Here's how the part is built. I have some questions about the finished solid (model axes, mm). Face numbers are marked on the shaded views. A direction names the side the tool comes from. Coordinates: 2 decimals unless noted, no trailing zeros. Write each loop counter-clockwise with the first axis right and the second up, starting at its lowest first coordinate (ties: lowest second). Pieces come first, ordered by that corner, then holes.
(1) For pin 1 Ø4 at (x, z) = (-41, 31) entering from +Y; pin 2 Ø2.5 at (x, y) = (39.5, -1) entering from +Z; pin 3 Ø5.5 at (y, z) = (4.5, 50.5) entering from -X, each with a flat end and sliding along its axis, tell me the tip position at first contact or that it passes through.
(2) Imagine slicing it at B-B, the plane z = 27.5. List the corners of the cut face in (x, y) for me.
(3) Which directions (+Z, -Z, +X, -X, +Y, -Y) give clear straight access to the entire face, cutting with the end or side of a thin tool? Please do the marked faces 1, 2, 3 and 4.
(4) Imagine slicing it at A-A, the plane y = 4.5. List the corners of the cut face in (x, z) for me.
(5) Imagine slicing it at C-C, the plane x = -28.5. List the corners of the cut face in (y, z) for me.
(6) Please list where these lines run through material, in increasing order: probe 1 along Z at (x, y) = (13.5, -5); probe 2 along X at (y, z) = (-6, 5.5); probe 3 along Y at (x, z) = (-12, 51).
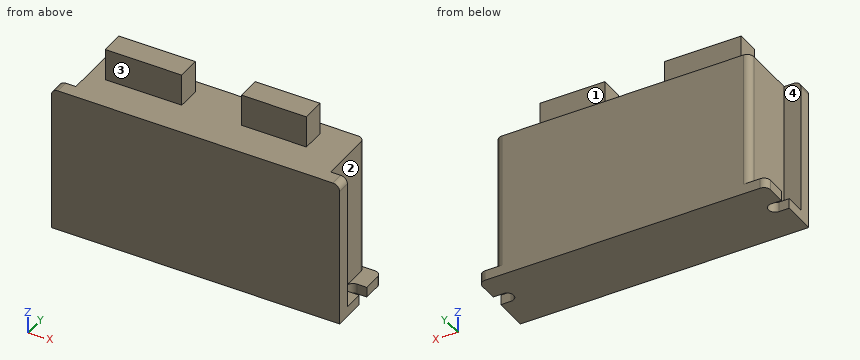
```python
from build123d import *

# Parameters (mm, degrees)
SKETCH1_W           = 86
SKETCH1_H           = 21.5
BOSS_EXTRUDE1_DEPTH = 43.75
SKETCH2_W           = 5
SKETCH2_H           = 17.5
CUT_EXTRUDE1_DEPTH  = 40.75
CUT_EXTRUDE2_DEPTH  = 63.278607884
FILLET1_R           = 2
SKETCH4_W           = 22.8
SKETCH4_H           = 7
SKETCH4_W_2         = 19.4
BOSS_EXTRUDE2_DEPTH = 9.5


with BuildPart() as part:
    # Sketch1 → Boss-Extrude1 (new body)
    with BuildSketch(Plane.XY):
        Rectangle(SKETCH1_W, SKETCH1_H)
    extrude(amount=BOSS_EXTRUDE1_DEPTH)

    # Sketch2 → Cut-Extrude1 (cut)
    with BuildSketch(Plane.XY.offset(43.75)):
        with Locations((-40.5, 2)):
            Rectangle(SKETCH2_W, SKETCH2_H)
        with Locations((40.5, 2)):
            Rectangle(SKETCH2_W, SKETCH2_H)
    extrude(amount=-CUT_EXTRUDE1_DEPTH, mode=Mode.SUBTRACT)

    # Sketch3 → Cut-Extrude2 (cut, through all)
    with BuildSketch(Plane(origin=(0, 0, 0), x_dir=(-1, 0, 0), z_dir=(0, 0, -1))):
        with BuildLine():
            Line((40, 3.25), (47.671145092, 3.25))
            ThreePointArc((47.671145092, 3.25), (49.671145092, 1.25), (47.671145092, -0.75))
            Line((47.671145092, -0.75), (40, -0.75))
            ThreePointArc((40, -0.75), (38, 1.25), (40, 3.25))
        make_face()
        with BuildLine():
            Line((-40, 3.25), (-47.671145092, 3.25))
            ThreePointArc((-47.671145092, 3.25), (-49.671145092, 1.25), (-47.671145092, -0.75))
            Line((-47.671145092, -0.75), (-40, -0.75))
            ThreePointArc((-40, -0.75), (-38, 1.25), (-40, 3.25))
        make_face()
    extrude(amount=-CUT_EXTRUDE2_DEPTH, mode=Mode.SUBTRACT)

    # Fillet1
    fillet1_edges = [part.edges().sort_by_distance(p)[0] for p in [
        (-43, -8.75, 43.75),
        (-43, 10.75, 1.5),
        (43, 10.75, 1.5),
        (-38, 10.75, 23.375),
        (38, 10.75, 23.375),
        (43, -8.75, 43.75),
    ]]
    fillet(fillet1_edges, radius=FILLET1_R)

    # Sketch4 → Boss-Extrude2 (add)
    with BuildSketch(Plane.XY.offset(43.75)):
        with Locations((-21.6, 3.25)):
            Rectangle(SKETCH4_W, SKETCH4_H)
        with Locations((17.3, 3.25)):
            Rectangle(SKETCH4_W_2, SKETCH4_H)
    extrude(amount=BOSS_EXTRUDE2_DEPTH)


solid = part.part
```
Recorded:
1. pin 1: stops at y = -6.75
1. pin 2: stops at z = 3
1. pin 3: stops at x = -33
2. outline: (-43, -10.75) - (43, -10.75) - (43, -6.75) - (38, -6.75) - (38, 8.75) arc R2 ccw to (36, 10.75) - (-36, 10.75) arc R2 ccw to (-38, 8.75) - (-38, -6.75) - (-43, -6.75) - close
3. face 1: +Z, +X, -X, +Y
3. face 2: +Z, +X, +Y
3. face 3: +Z, +X, -X, -Y
3. face 4: +Z, -X, +Y
4. outline: (-43, 0) - (43, 0) - (43, 3) - (38, 3) - (38, 43.75) - (27, 43.75) - (27, 53.25) - (7.6, 53.25) - (7.6, 43.75) - (-10.2, 43.75) - (-10.2, 53.25) - (-33, 53.25) - (-33, 43.75) - (-38, 43.75) - (-38, 3) - (-43, 3) - close
5. outline: (-10.75, 0) - (10.75, 0) - (10.75, 43.75) - (6.75, 43.75) - (6.75, 53.25) - (-0.25, 53.25) - (-0.25, 43.75) - (-10.75, 43.75) - close
6. probe 1: z = 0 to 43.75
6. probe 2: x = -38 to 38
6. probe 3: y = -0.25 to 6.75
